Could you check a few things on this model? Use its own coordinates, in mm. Face numbers are marked on the shaded views. A direction names the side the tool comes from. Coordinates: 2 decimals unless noted, no trailing zeros. Order: outer loops, then holes, each group sorted by start corner. A loop starts at its lowest first (then second) coordinate and runs counter-clockwise, first axis right, second up. Notation, with made-up numbers: (-12.75, 62.25) - (42.25, 62.25) arc R26 ccw to (42.25, 96.25) - close; hole circle Ø10 at (8, 38.25). An arc over 180 degrees is marked (long way). Answer as CSV lines item,"result". Start each with the question number.
1. I want a section at C-C, the plane y = -8. List the corners of the cut face in (x, z) for me, and give its area (3 significant figures).
2. Thinking about a two-plate mould opening in X: for the marked faces 1, 2 and 3, which applies, released by +X, released by -X, zero draft, split by the parting line, or undercut?
3. For the marked faces 4, 5 and 6, which set-ups out of +Z, -Z, +X, -X, +Y, -Y let a thin tool reach every point of the face, with its end or its side?
4. I want a section at B-B, the plane x = 25. List the corners of the cut face in (y, z) for me.
5. I need wall thicknesses on probe 1 along Y at (x, z) = (25, 11); probe 2 along Y at (x, z) = (1.5, -21); probe 3 along X at (y, z) = (-12, 17). Which ranges of each line are inside material? Lowest first, please.
6. For pin 1 (9.5 mm diameter, centred on x = 21, y = 8.5, fed in from -Z); pin 2 (18.5 mm diameter, centred on y = 0.5, z = -28.5, fed in from -X); pin 3 (10 mm diameter, centred on x = -13, z = -31, fed in from -Y); pin 4 (4 mm diameter, centred on x = 31, y = 11.5, fed in from +Z), each with a flat end and sliding along its axis, tell me the tip position at first contact or that it passes through.
7. I want a section at A-A, the plane z = 16. List the corners of the cut face in (x, y) for me, and give its area (3 significant figures).
8. I want a section at D-D, the plane y = 5. List the corners of the cut face in (x, z) for me, and give its area (3 significant figures).
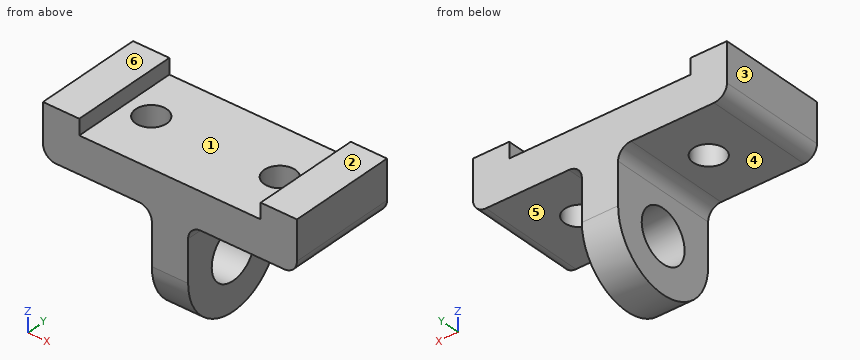
from build123d import *

# Parameters (mm, degrees)
SKETCH1_W           = 98
SKETCH1_H           = 42
BOSS_EXTRUDE1_DEPTH = 14
SKETCH3_R           = 6
CUT_EXTRUDE1_DEPTH  = 31
SKETCH3_3_R         = 6
CUT_EXTRUDE2_DEPTH  = 150
FILLET1_R           = 5
SKETCH4_W           = 14
SKETCH4_H           = 42
BOSS_EXTRUDE2_DEPTH = 6
FILLET2_R           = 5
SKETCH5_W           = 14
SKETCH5_H           = 42
BOSS_EXTRUDE3_DEPTH = 6
SKETCH6_W           = 42
SKETCH6_H           = 42
BOSS_EXTRUDE4_DEPTH = 7
FILLET4_RADIUS      = 21
FILLET4_LENGTH      = 14
SKETCH7_R           = 10
CUT_EXTRUDE3_DEPTH  = 20.5
FILLET5_R           = 5


with BuildPart() as part:
    # Sketch1 → Boss-Extrude1 (new body)
    with BuildSketch(Plane.XY):
        Rectangle(SKETCH1_W, SKETCH1_H)
    extrude(amount=BOSS_EXTRUDE1_DEPTH)

    # Sketch3 → Cut-Extrude1 (cut)
    with BuildSketch(Plane.XY):
        with Locations(Location((25, 0, 0), (0, 0, 180))):
            Circle(SKETCH3_R)
    extrude(amount=CUT_EXTRUDE1_DEPTH, mode=Mode.SUBTRACT)

    # Sketch3<3> → Cut-Extrude2 (cut)
    with BuildSketch(Plane.XY):
        with Locations(Location((-25, 0.49893218, 0), (0, 0, 180))):
            Circle(SKETCH3_3_R)
        with Locations(Location((25, 0, 0), (0, 0, 180))):
            Circle(SKETCH3_3_R)
    extrude(amount=CUT_EXTRUDE2_DEPTH, mode=Mode.SUBTRACT)

    # Fillet1
    fillet1_edges = [part.edges().sort_by_distance(p)[0] for p in [
        (-49, 0, 0),
    ]]
    fillet(fillet1_edges, radius=FILLET1_R)

    # Sketch4 → Boss-Extrude2 (add)
    with BuildSketch(Plane.XY.offset(14)):
        with Locations((-42, 0)):
            Rectangle(SKETCH4_W, SKETCH4_H)
    extrude(amount=BOSS_EXTRUDE2_DEPTH)

    # Fillet2
    fillet2_edges = [part.edges().sort_by_distance(p)[0] for p in [
        (49, 0, 0),
    ]]
    fillet(fillet2_edges, radius=FILLET2_R)

    # Sketch5 → Boss-Extrude3 (add)
    with BuildSketch(Plane.XY.offset(14)):
        with Locations((42, 0)):
            Rectangle(SKETCH5_W, SKETCH5_H)
    extrude(amount=BOSS_EXTRUDE3_DEPTH)

    # Sketch6 → Boss-Extrude4 (add, symmetric)
    with BuildSketch(Plane(origin=(0, 0, 0), x_dir=(0, 0, -1), z_dir=(1, 0, 0))):
        with Locations((21, 0)):
            Rectangle(SKETCH6_W, SKETCH6_H)
    extrude(amount=BOSS_EXTRUDE4_DEPTH, both=True)

    # Fillet4: full round fillet: the end face becomes a half cylinder, R = half its width
    fillet4_face = Plane((0, 0, -42), x_dir=(-1, 0, 0), z_dir=(0, 0, -1))  # on the end face: x along it, z out of the body
    fillet4_slab = fillet4_face.offset(-FILLET4_RADIUS / 2) * Box(FILLET4_LENGTH, 2 * FILLET4_RADIUS, FILLET4_RADIUS, mode=Mode.PRIVATE)  # the body's end, R deep
    fillet4_round = Plane((0, 0, -21), x_dir=(0, 0, -1), z_dir=(-1, 0, 0)) * Cylinder(FILLET4_RADIUS, FILLET4_LENGTH, mode=Mode.PRIVATE)  # its axis R under the face
    add(fillet4_slab - fillet4_round, mode=Mode.SUBTRACT)

    # Sketch7 → Cut-Extrude3 (cut, symmetric)
    with BuildSketch(Plane(origin=(0, 0, 0), x_dir=(0, 0, -1), z_dir=(1, 0, 0))):
        with Locations((21, 0)):
            Circle(SKETCH7_R)
    extrude(amount=CUT_EXTRUDE3_DEPTH, both=True, mode=Mode.SUBTRACT)

    # Fillet5
    fillet5_edges = [part.edges().sort_by_distance(p)[0] for p in [
        (-7, 0, 0),
        (7, 0, 0),
    ]]
    fillet(fillet5_edges, radius=FILLET5_R)


solid = part.part
Solved:
1,outline,"(-49, 5) arc R5 ccw to (-44, 0) - (-12, 0) arc R5 cw to (-7, -5) - (-7, -15) - (7, -15) - (7, -5) arc R5 cw to (12, 0) - (44, 0) arc R5 ccw to (49, 5) - (49, 20) - (35, 20) - (35, 14) - (-35, 14) - (-35, 20) - (-49, 20) - close; (-7, -40.42) - (7, -40.42) - (7, -27) - (-7, -27) - close"
1,area,"1,940 mm2"
2,face 1,"undercut"
2,face 2,"zero draft"
2,face 3,"released by -X"
3,face 4,"-Z, -X, +Y, -Y"
3,face 5,"-Z, +X, +Y, -Y"
3,face 6,"+Z, +X, -X, +Y, -Y"
4,outline,"(-21, 0) - (-6, 0) - (-6, 14) - (-21, 14) - close; (6, 0) - (21, 0) - (21, 14) - (6, 14) - close"
5,probe 1,"y = -21 to -6, 6 to 21"
5,probe 2,"y = -21 to -10, 10 to 21"
5,probe 3,"x = -49 to -35, 35 to 49"
6,pin 1,"stops at z = 0"
6,pin 2,"stops at x = -7"
6,pin 3,"passes through"
6,pin 4,"stops at z = 14"
7,outline,"(-49, -21) - (-35, -21) - (-35, 21) - (-49, 21) - close; (35, -21) - (49, -21) - (49, 21) - (35, 21) - close"
7,area,"1,180 mm2"
8,outline,"(-49, 5) arc R5 ccw to (-44, 0) - (-28.97, 0) - (-28.97, 14) - (-35, 14) - (-35, 20) - (-49, 20) - close; (-21.03, 0) - (-12, 0) arc R5 cw to (-7, -5) - (-7, -12.34) - (7, -12.34) - (7, -5) arc R5 cw to (12, 0) - (21.68, 0) - (21.68, 14) - (-21.03, 14) - close; (-7, -41.4) - (7, -41.4) - (7, -29.66) - (-7, -29.66) - close; (28.32, 0) - (44, 0) arc R5 ccw to (49, 5) - (49, 20) - (35, 20) - (35, 14) - (28.32, 14) - close"
8,area,"1,670 mm2"
